For this review, take the finished solid that the model builds, in its own axes (mm). Round coordinates to 2 decimals unless told otherwise and drop trailing zeros.
1) Insertion check: pin 1 (2.5 mm diameter, centred on x = 76, y = 4.5, fed in from +Z); pin 2 (0.9 mm diameter, centred on x = 162, y = 3.5, fed in from +Z); pin 3 (3 mm diameter, centred on y = 3, z = 8, fed in from -X). Each pin has a flat end and moves straight along its axis. Give the tip position at first contact, or say it passes through.
2) Take a section at A-A (z = 7). Give the number of separate pieces and of enclosed holes in the cut face, then the cut area to 3 significant figures.
3) Wall thickness on L1, parallel to Z at x = 177, y = 6.5: over which ranges is the line inside the solid? List them lowest first.
4) Mouldability with a two-part tool opening along X and no side actions: class faces 1 (the flat face through (0, 4, 2)), 2 (the flat face through (118, 4, 7)), 3 (the flat face through (98, 4, 7)), 4 (the flat face through (99, 7.5, 4)) as pulls with the +X half, pulls with the -X half, needs draft (parallel to the pull), parting line crosses it, or undercut.
```python
from build123d import *

# Parameters (mm, degrees)
F0_W     = 3
F0_H     = 7.5
F1_DEPTH = 3.5
F0_W_2   = 2
F2_DEPTH = 10


with BuildPart() as f1:
    # F0 (on Top) → F1 (new body)
    with BuildSketch(Plane.XY):
        with Locations((1.5, 3.75)):
            Rectangle(F0_W, F0_H)
        with Locations((6.5, 3.75)):
            Rectangle(F0_W, F0_H)
        with Locations((11.5, 3.75)):
            Rectangle(F0_W, F0_H)
        with Locations((16.5, 3.75)):
            Rectangle(F0_W, F0_H)
        with Locations((21.5, 3.75)):
            Rectangle(F0_W, F0_H)
        with Locations((26.5, 3.75)):
            Rectangle(F0_W, F0_H)
        with Locations((31.5, 3.75)):
            Rectangle(F0_W, F0_H)
        with Locations((36.5, 3.75)):
            Rectangle(F0_W, F0_H)
        with Locations((41.5, 3.75)):
            Rectangle(F0_W, F0_H)
        with Locations((46.5, 3.75)):
            Rectangle(F0_W, F0_H)
        with Locations((51.5, 3.75)):
            Rectangle(F0_W, F0_H)
        with Locations((56.5, 3.75)):
            Rectangle(F0_W, F0_H)
        with Locations((61.5, 3.75)):
            Rectangle(F0_W, F0_H)
        with Locations((66.5, 3.75)):
            Rectangle(F0_W, F0_H)
        with Locations((71.5, 3.75)):
            Rectangle(F0_W, F0_H)
        with Locations((76.5, 3.75)):
            Rectangle(F0_W, F0_H)
        with Locations((81.5, 3.75)):
            Rectangle(F0_W, F0_H)
        with Locations((86.5, 3.75)):
            Rectangle(F0_W, F0_H)
        with Locations((91.5, 3.75)):
            Rectangle(F0_W, F0_H)
        with Locations((96.5, 3.75)):
            Rectangle(F0_W, F0_H)
        with Locations((101.5, 3.75)):
            Rectangle(F0_W, F0_H)
        with Locations((106.5, 3.75)):
            Rectangle(F0_W, F0_H)
        with Locations((111.5, 3.75)):
            Rectangle(F0_W, F0_H)
        with Locations((116.5, 3.75)):
            Rectangle(F0_W, F0_H)
        with Locations((121.5, 3.75)):
            Rectangle(F0_W, F0_H)
        with Locations((126.5, 3.75)):
            Rectangle(F0_W, F0_H)
        with Locations((131.5, 3.75)):
            Rectangle(F0_W, F0_H)
        with Locations((136.5, 3.75)):
            Rectangle(F0_W, F0_H)
        with Locations((141.5, 3.75)):
            Rectangle(F0_W, F0_H)
        with Locations((146.5, 3.75)):
            Rectangle(F0_W, F0_H)
        with Locations((151.5, 3.75)):
            Rectangle(F0_W, F0_H)
        with Locations((156.5, 3.75)):
            Rectangle(F0_W, F0_H)
        with Locations((161.5, 3.75)):
            Rectangle(F0_W, F0_H)
        with Locations((166.5, 3.75)):
            Rectangle(F0_W, F0_H)
        with Locations((171.5, 3.75)):
            Rectangle(F0_W, F0_H)
        with Locations((176.5, 3.75)):
            Rectangle(F0_W, F0_H)
        with Locations((181.5, 3.75)):
            Rectangle(F0_W, F0_H)
        with Locations((186.5, 3.75)):
            Rectangle(F0_W, F0_H)
        with Locations((191.5, 3.75)):
            Rectangle(F0_W, F0_H)
        with Locations((196.5, 3.75)):
            Rectangle(F0_W, F0_H)
    extrude(amount=F1_DEPTH)

    # F0 (on Top) → F2 (join)
    with BuildSketch(Plane.XY):
        with Locations((4, 3.75)):
            Rectangle(F0_W_2, F0_H)
        with Locations((9, 3.75)):
            Rectangle(F0_W_2, F0_H)
        with Locations((14, 3.75)):
            Rectangle(F0_W_2, F0_H)
        with Locations((19, 3.75)):
            Rectangle(F0_W_2, F0_H)
        with Locations((24, 3.75)):
            Rectangle(F0_W_2, F0_H)
        with Locations((29, 3.75)):
            Rectangle(F0_W_2, F0_H)
        with Locations((34, 3.75)):
            Rectangle(F0_W_2, F0_H)
        with Locations((39, 3.75)):
            Rectangle(F0_W_2, F0_H)
        with Locations((44, 3.75)):
            Rectangle(F0_W_2, F0_H)
        with Locations((49, 3.75)):
            Rectangle(F0_W_2, F0_H)
        with Locations((54, 3.75)):
            Rectangle(F0_W_2, F0_H)
        with Locations((59, 3.75)):
            Rectangle(F0_W_2, F0_H)
        with Locations((64, 3.75)):
            Rectangle(F0_W_2, F0_H)
        with Locations((69, 3.75)):
            Rectangle(F0_W_2, F0_H)
        with Locations((74, 3.75)):
            Rectangle(F0_W_2, F0_H)
        with Locations((79, 3.75)):
            Rectangle(F0_W_2, F0_H)
        with Locations((84, 3.75)):
            Rectangle(F0_W_2, F0_H)
        with Locations((89, 3.75)):
            Rectangle(F0_W_2, F0_H)
        with Locations((94, 3.75)):
            Rectangle(F0_W_2, F0_H)
        with Locations((99, 3.75)):
            Rectangle(F0_W_2, F0_H)
        with Locations((104, 3.75)):
            Rectangle(F0_W_2, F0_H)
        with Locations((109, 3.75)):
            Rectangle(F0_W_2, F0_H)
        with Locations((114, 3.75)):
            Rectangle(F0_W_2, F0_H)
        with Locations((119, 3.75)):
            Rectangle(F0_W_2, F0_H)
        with Locations((124, 3.75)):
            Rectangle(F0_W_2, F0_H)
        with Locations((129, 3.75)):
            Rectangle(F0_W_2, F0_H)
        with Locations((134, 3.75)):
            Rectangle(F0_W_2, F0_H)
        with Locations((139, 3.75)):
            Rectangle(F0_W_2, F0_H)
        with Locations((144, 3.75)):
            Rectangle(F0_W_2, F0_H)
        with Locations((149, 3.75)):
            Rectangle(F0_W_2, F0_H)
        with Locations((154, 3.75)):
            Rectangle(F0_W_2, F0_H)
        with Locations((159, 3.75)):
            Rectangle(F0_W_2, F0_H)
        with Locations((164, 3.75)):
            Rectangle(F0_W_2, F0_H)
        with Locations((169, 3.75)):
            Rectangle(F0_W_2, F0_H)
        with Locations((174, 3.75)):
            Rectangle(F0_W_2, F0_H)
        with Locations((179, 3.75)):
            Rectangle(F0_W_2, F0_H)
        with Locations((184, 3.75)):
            Rectangle(F0_W_2, F0_H)
        with Locations((189, 3.75)):
            Rectangle(F0_W_2, F0_H)
        with Locations((194, 3.75)):
            Rectangle(F0_W_2, F0_H)
        with Locations((199, 3.75)):
            Rectangle(F0_W_2, F0_H)
    extrude(amount=F2_DEPTH)


solid = f1.part
```
Response:
1. pin 1: stops at z = 10
1. pin 2: stops at z = 3.5
1. pin 3: stops at x = 3
2. separate pieces: 40
2. enclosed holes: 0
2. area: 600 mm2
3. L1: z = 0 to 3.5
4. face 1: pulls with the -X half
4. face 2: undercut
4. face 3: undercut
4. face 4: needs draft
